from build123d import *

# Parameters (mm, degrees)
BOSS_EXTRUDE1_DEPTH = 65.8876
BOSS_EXTRUDE2_DEPTH = 29.3624
SKETCH4_R           = 2
BOSS_EXTRUDE3_DEPTH = 15.4559
FILLET1_R           = 1.27


with BuildPart() as part:
    # Sketch1 → Boss-Extrude1 (new body)
    with BuildSketch(Plane(origin=(0, 0, 0), x_dir=(1, 0, 0), z_dir=(0, 1, 0))):
        with BuildLine():
            Line((-12.2809, 0), (-15.4559, 0))
            Line((-15.4559, 0), (-15.4559, -15.4559))
            Line((-15.4559, -15.4559), (0, -15.4559))
            Line((0, -15.4559), (15.4559, -15.4559))
            Line((15.4559, -15.4559), (15.4559, 0))
            Line((15.4559, 0), (12.2809, 0))
            ThreePointArc((12.2809, 0), (0, -12.2809), (-12.2809, 0))
        make_face()
    extrude(amount=BOSS_EXTRUDE1_DEPTH)

    # Sketch2 → Boss-Extrude2 (add)
    with BuildSketch(Plane(origin=(0, 65.8876, 0), x_dir=(1, 0, 0), z_dir=(0, 1, 0))):
        Polygon((-12.2809, -12.2809), (0, -12.2809), (12.2809, -12.2809), (15.4559, -12.2809), (15.4559, -15.4559), (-15.4559, -15.4559), (-15.4559, -12.2809), align=None)
    boss_extrude2 = extrude(amount=BOSS_EXTRUDE2_DEPTH)

    # Mirror1: Boss-Extrude2 across plane
    add(boss_extrude2.mirror(Plane.ZX.offset(32.9438)))

    # Sketch4 → Boss-Extrude3 (add, through all)
    # profile 1 of 6: a face of its own
    with BuildSketch(Plane(origin=(0, 0, 0), x_dir=(-1, 0, 0), z_dir=(0, 0, -1))):
        with BuildLine():
            Line((-15.4559, 39.2938), (-15.4559, 26.5938))
            Line((-15.4559, 26.5938), (-18.6309, 26.5938))
            ThreePointArc((-18.6309, 26.5938), (-24.9809, 32.9438), (-18.6309, 39.2938))
            Line((-18.6309, 39.2938), (-15.4559, 39.2938))
        make_face()
        with Locations((-18.6309, 32.9438)):
            Circle(SKETCH4_R, mode=Mode.SUBTRACT)
    # profile 2 of 6: a face of its own
    with BuildSketch(Plane(origin=(0, 0, 0), x_dir=(-1, 0, 0), z_dir=(0, 0, -1))):
        with BuildLine():
            Line((-15.4559, 12.7), (-18.6309, 12.7))
            ThreePointArc((-18.6309, 12.7), (-24.9809, 6.35), (-18.6309, 0))
            Line((-18.6309, 0), (-15.4559, 0))
            Line((-15.4559, 0), (-15.4559, 12.7))
        make_face()
        with Locations(Location((-18.6309, 6.35, 0), (0, 0, 180))):
            Circle(SKETCH4_R, mode=Mode.SUBTRACT)
    # profile 3 of 6: a face of its own
    with BuildSketch(Plane(origin=(0, 0, 0), x_dir=(-1, 0, 0), z_dir=(0, 0, -1))):
        with BuildLine():
            Line((-18.6309, 65.8876), (-15.4559, 65.8876))
            Line((-15.4559, 65.8876), (-15.4559, 53.1876))
            Line((-15.4559, 53.1876), (-18.6309, 53.1876))
            ThreePointArc((-18.6309, 53.1876), (-24.9809, 59.5376), (-18.6309, 65.8876))
        make_face()
        with Locations((-18.6309, 59.5376)):
            Circle(SKETCH4_R, mode=Mode.SUBTRACT)
    # profile 4 of 6: a face of its own
    with BuildSketch(Plane(origin=(0, 0, 0), x_dir=(-1, 0, 0), z_dir=(0, 0, -1))):
        with BuildLine():
            Line((18.6309, 0), (15.4559, 0))
            Line((15.4559, 0), (15.4559, 12.7))
            Line((15.4559, 12.7), (18.6309, 12.7))
            ThreePointArc((18.6309, 12.7), (24.9809, 6.35), (18.6309, 0))
        make_face()
        with Locations((18.6309, 6.35)):
            Circle(SKETCH4_R, mode=Mode.SUBTRACT)
    # profile 5 of 6: a face of its own
    with BuildSketch(Plane(origin=(0, 0, 0), x_dir=(-1, 0, 0), z_dir=(0, 0, -1))):
        with BuildLine():
            Line((15.4559, 53.1876), (18.6309, 53.1876))
            ThreePointArc((18.6309, 53.1876), (24.9809, 59.5376), (18.6309, 65.8876))
            Line((18.6309, 65.8876), (15.4559, 65.8876))
            Line((15.4559, 65.8876), (15.4559, 53.1876))
        make_face()
        with Locations(Location((18.6309, 59.5376, 0), (0, 0, 180))):
            Circle(SKETCH4_R, mode=Mode.SUBTRACT)
    # profile 6 of 6: a face of its own
    with BuildSketch(Plane(origin=(0, 0, 0), x_dir=(-1, 0, 0), z_dir=(0, 0, -1))):
        with BuildLine():
            Line((18.6309, 26.5938), (15.4559, 26.5938))
            Line((15.4559, 26.5938), (15.4559, 39.2938))
            Line((15.4559, 39.2938), (18.6309, 39.2938))
            ThreePointArc((18.6309, 39.2938), (24.9809, 32.9438), (18.6309, 26.5938))
        make_face()
        with Locations(Location((18.6309, 32.9438, 0), (0, 0, 180))):
            Circle(SKETCH4_R, mode=Mode.SUBTRACT)
    extrude(amount=-BOSS_EXTRUDE3_DEPTH)

    # Fillet1
    fillet1_edges = [part.edges().sort_by_distance(p)[0] for p in [
        (-15.4559, 0, 13.8684),
        (-15.4559, 95.25, 13.8684),
        (15.4559, 95.25, 13.8684),
        (15.4559, -29.3624, 13.8684),
        (-15.4559, -29.3624, 13.8684),
        (15.4559, 65.8876, 13.8684),
        (15.4559, 0, 13.8684),
        (-15.4559, 65.8876, 13.8684),
    ]]
    fillet(fillet1_edges, radius=FILLET1_R)


solid = part.part
Verification items for the finished model (mm, model axes). A direction names the side the tool comes from. Give positions to 0.01 mm unless a question says otherwise; leave off trailing zeros. Loops run counter-clockwise (first coordinate to the right, second up) from the corner with the lowest first, then second, coordinate; pieces in that order, holes last. Notation, with made-up numbers: (35.25, 1) - (54.25, 1) arc R13 ccw to (54.25, 18) - close; hole circle Ø9 at (-3.75, -2). An arc over 180 degrees is marked (long way). Write item = value, one per line. Start each with the question number.
Q1. Tool access check on faces 1 (the face through (0, -14, 12.281)), 2 (the face through (-17, 53.188, 8)), 3 (the face through (-15.456, -14, 14)), 4 (the face through (15.456, 20, 8)). Record the directions out of +Z, -Z, +X, -X, +Y, -Y that give a thin tool (end or side, any length) a straight path to the whole face; none if there is none.
Q2. Cross-section at C-C, the plane x = -6. Enter the section's corners in (y, z).
Q3. Cross-section at A-A, the plane y = 6.35. Enter the section's corners in (x, z), and give its area (3 significant figures).
Q4. Cross-section at D-D, the plane y = 48. Enter the section's corners in (x, z), and give its area (3 significant figures).
Q5. Mould release check, pull along Y, two halves, no side actions. Record for faces 5 (the face through (0, 80, 12.281)), 6 (the face through (0, -29.362, 14)), 7 (the face through (-17, 39.294, 8)), 8 (the face through (24.98, 6.49, 7.62)): released by +Y, released by -Y, zero draft, split by the parting line, or undercut.
Q6. Cross-section at B-B, the plane z = 2.5. State how many separate pieces and enclosed holes the cut face has, and give its area (3 significant figures).
Q7. Depth check by flat-ended pin: P1, Ø4.5, axis at x = 11, z = 6.5, coming from the +Y side; P2, Ø14.5, axis at x = -1.5, y = 79.5, coming from the -Z side; P3, Ø12, axis at x = 1.5, y = 70, coming from the -Z side; P4, Ø3.5, axis at x = -18.63, y = 59.54, coming from the +Z side. Enter the tip coordinate at first touch or a pass-through.
Q8. Thickness scan on line 1 (Y direction, x = -18.5, z = 2.5); line 2 (Y direction, x = -16.5, z = 1); line 3 (Y direction, x = 18, z = 14.5). Record the ranges inside material, lowest first.
Answer key:
q1.face_1 = -Z, +X, -X, -Y
q1.face_2 = +Z, -Z, -X
q1.face_3 = +Z, -Z, -X, -Y
q1.face_4 = +Z, -Z, +X
q2.outline = (-29.36, 12.28) - (0, 12.28) - (0, 10.72) - (65.89, 10.72) - (65.89, 12.28) - (95.25, 12.28) - (95.25, 15.46) - (-29.36, 15.46) - close
q3.outline = (-24.98, 0) - (-20.63, 0) - (-20.63, 15.46) - (-24.98, 15.46) - close; (-16.63, 0) - (-12.28, 0) arc R12.28 cw to (12.28, 0) - (16.63, 0) - (16.63, 15.46) - (-16.63, 15.46) - close; (20.63, 0) - (24.98, 0) - (24.98, 15.46) - (20.63, 15.46) - close
q3.area = 412 mm^2
q4.outline = (-15.46, 0) - (-12.28, 0) arc R12.28 cw to (12.28, 0) - (15.46, 0) - (15.46, 15.46) - (-15.46, 15.46) - close
q4.area = 241 mm^2
q5.face_5 = zero draft
q5.face_6 = released by -Y
q5.face_7 = undercut
q5.face_8 = undercut
q6.separate_pieces = 2
q6.enclosed_holes = 6
q6.area = 999 mm^2
q7.P1 = 65.89
q7.P2 = 12.28
q7.P3 = 10.79
q7.P4 = through
q8.line_1 = 0 to 4.35, 8.35 to 12.7, 26.59 to 30.95, 34.94 to 39.29, 53.19 to 57.54, 61.53 to 65.89
q8.line_2 = 0 to 12.7, 26.59 to 39.29, 53.19 to 65.89
q8.line_3 = 0 to 4.45, 8.25 to 12.7, 26.59 to 31.05, 34.84 to 39.29, 53.19 to 57.64, 61.44 to 65.89
